Autodesk Inventor part; units mm, degrees
ref_plane "YZ Plane" through (0, 0, 0) normal (1, 0, 0) x (0, 1, 0)
ref_plane "XZ Plane" through (0, 0, 0) normal (0, 1, 0) x (-1, 0, 0)
ref_plane "XY Plane" through (0, 0, 0) normal (0, 0, 1) x (1, 0, 0)
sketch "Sketch1" plane through (0, 0, 0) normal (0, 0, 1) x (1, 0, 0)
  line L0 (3.6, -16) -> (3.6, 16)
  line L1 (-3.6, 16) -> (-3.6, -16)
  arc A0 (3.6, 16) -> (-3.6, 16) centre (0, 16) ccw
  circle A1 centre (0, 8) radius 2.4
  circle A2 centre (0, 8) radius 3.2
  circle A3 centre (0, 0) radius 3.2
  circle A4 centre (0, 0) radius 2.4
  line L2 (0, 0) -> (0, 8) construction
  line L3 (-2.8, 5.7373) -> (-2.8, 2.2627)
  line L4 (2.8, 5.7373) -> (2.8, 2.2627)
  arc A5 (-2.8, 5.7373) -> (2.8, 5.7373) centre (0, 8) ccw
  arc A6 (2.8, 2.2627) -> (-2.8, 2.2627) centre (0, 0) ccw
  arc A7 (-3.6, -16) -> (3.6, -16) centre (0, -16) ccw
  circle A8 centre (0, -8) radius 3.2
  circle A9 centre (0, -8) radius 2.4
  line L5 (0, 0) -> (0, -8) construction
  line L6 (-2.8, -2.2627) -> (-2.8, -5.7373)
  line L7 (2.8, -2.2627) -> (2.8, -5.7373)
  arc A10 (-2.8, -2.2627) -> (2.8, -2.2627) centre (0, 0) ccw
  arc A11 (2.8, -5.7373) -> (-2.8, -5.7373) centre (0, -8) ccw
  circle A12 centre (0, 16) radius 3.2
  circle A13 centre (0, 16) radius 2.4
  circle A14 centre (0, -16) radius 3.2
  circle A15 centre (0, -16) radius 2.4
  line L8 (0, 16) -> (0, 8) construction
  line L9 (0, -8) -> (0, -16) construction
  line L10 (2.8, 13.7373) -> (2.8, 10.2627)
  line L11 (-2.8, 13.7373) -> (-2.8, 10.2627)
  arc A16 (-2.8, 13.7373) -> (2.8, 13.7373) centre (0, 16) ccw
  arc A17 (2.8, 10.2627) -> (-2.8, 10.2627) centre (0, 8) ccw
  arc A18 (-2.8, -10.2627) -> (2.8, -10.2627) centre (0, -8) ccw
  arc A19 (2.8, -13.7373) -> (-2.8, -13.7373) centre (0, -16) ccw
  line L12 (2.8, -13.7373) -> (2.8, -10.2627)
  line L13 (-2.8, -10.2627) -> (-2.8, -13.7373)
  dimension "d8" = 4.8
  dimension "d9" = 6.4
  dimension "d32" = 7.2
  dimension "d34" = 8
  dimension "d36" = 0.8
extrude "Extrusion1" add sketch "Sketch1" along normal mid plane 8 contours A7 L1 A0 L0 | A2 | A3 | A5 L4 A6 L3 | A8 | A10 L7 A11 L6 | A12 | A14 | L10 A17 L11 A16 | A18 L12 A19 L13
sketch "Sketch6" plane through (0, 0, 4) normal (0, 0, 1) x (1, 0, 0)
  circle A0 centre (0, 0) radius 2.4
  circle A1 centre (0, 8) radius 2.4
  circle A2 centre (0, 0) radius 3.2
  circle A3 centre (0, 8) radius 3.2
  arc A4 (2.8, 2.2627) -> (-2.8, 2.2627) centre (0, 0) ccw
  line L0 (-2.8, 5.7373) -> (-2.8, 2.2627)
  arc A5 (-2.8, 5.7373) -> (2.8, 5.7373) centre (0, 8) ccw
  line L1 (2.8, 5.7373) -> (2.8, 2.2627)
  line L2 (-2.8, -2.2627) -> (-2.8, -5.7373)
  arc A6 (-2.8, -2.2627) -> (2.8, -2.2627) centre (0, 0) ccw
  arc A7 (2.8, -5.7373) -> (-2.8, -5.7373) centre (0, -8) ccw
  line L3 (2.8, -2.2627) -> (2.8, -5.7373)
  circle A8 centre (0, -8) radius 3.2
  circle A9 centre (0, -8) radius 2.4
  circle A10 centre (0, -16) radius 2.4
  circle A11 centre (0, 16) radius 2.4
  line L4 (2.8, -13.7373) -> (2.8, -10.2627)
  arc A12 (2.8, -13.7373) -> (-2.8, -13.7373) centre (0, -16) ccw
  arc A13 (-2.8, -10.2627) -> (2.8, -10.2627) centre (0, -8) ccw
  line L5 (-2.8, -10.2627) -> (-2.8, -13.7373)
  circle A14 centre (0, -16) radius 3.2
  circle A15 centre (0, 16) radius 3.2
  line L6 (2.8, 13.7373) -> (2.8, 10.2627)
  arc A16 (-2.8, 13.7373) -> (2.8, 13.7373) centre (0, 16) ccw
  arc A17 (2.8, 10.2627) -> (-2.8, 10.2627) centre (0, 8) ccw
  line L7 (-2.8, 13.7373) -> (-2.8, 10.2627)
extrude "Extrusion7" cut sketch "Sketch6" against normal blind 0.8 contours A2 | A3 | A8 | A14 | A15
extrude "Extrusion8" cut sketch "Sketch6" against normal blind 3.1 contours A4 L0 A5 L1 | A6 L3 A7 L2 | A12 L5 A13 L4 | L6 A17 L7 A16
mirror "Mirror1" about plane through (0, 0, 0) normal (0, 0, 1) of "Extrusion7", "Extrusion8"
fillet "Fillet1" radius 0.4 32 edges at (-2.8, 2.2627, 2.45) (-2.8, 5.7373, 2.45) (2.8, 2.2627, 2.45) (2.8, 5.7373, 2.45) (2.8, 5.7373, -2.45) (2.8, 2.2627, -2.45) (-2.8, 2.2627, -2.45) (-2.8, 5.7373, -2.45) (-2.8, -2.2627, 2.45) (-2.8, -5.7373, 2.45) (2.8, -5.7373, 2.45) (2.8, -2.2627, 2.45) (2.8, -2.2627, -2.45) (2.8, -5.7373, -2.45) (-2.8, -5.7373, -2.45) (-2.8, -2.2627, -2.45) (-2.8, -13.7373, 2.45) (-2.8, -13.7373, -2.45) (-2.8, -10.2627, 2.45) (-2.8, -10.2627, -2.45) (2.8, -13.7373, 2.45) (2.8, -10.2627, 2.45) (2.8, -13.7373, -2.45) (2.8, -10.2627, -2.45) (-2.8, 10.2627, 2.45) (-2.8, 13.7373, 2.45) (-2.8, 10.2627, -2.45) (-2.8, 13.7373, -2.45) (2.8, 10.2627, 2.45) (2.8, 13.7373, 2.45) (2.8, 10.2627, -2.45) (2.8, 13.7373, -2.45)
fillet "Fillet1" radius 0.1 8 edges at (0, -19.6, 4) (-3.6, 0, 4) (0, 19.6, 4) (3.6, 0, 4) (0, 19.6, -4) (-3.6, 0, -4) (0, -19.6, -4) (3.6, 0, -4)
equation "\"lf\" = 0.1"
equation "\"tf\" = 0.4"
properties part number "32316-DkBluishGray" material "ABS Plastic"
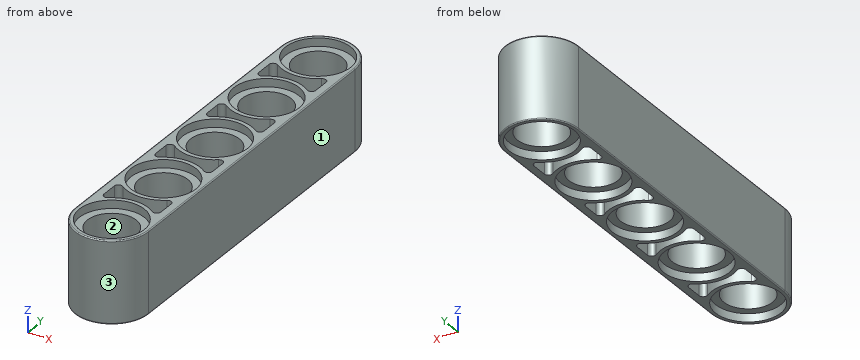
The model under review builds one solid part; all positions refer to its coordinate system, in mm. Face numbers are marked on the shaded views. Round coordinates to 2 decimals unless told otherwise and drop trailing zeros. Order: outer loops, then holes, each group sorted by start corner. A loop starts at its lowest first (then second) coordinate and runs counter-clockwise, first axis right, second up.
Item 1: For pin 1 (0.7 mm diameter, centred on x = 0.5, y = 12, fed in from +Z); pin 2 (3 mm diameter, centred on x = -1, y = -7, fed in from +Z); pin 3 (3 mm diameter, centred on x = -1, y = -7, fed in from -Z), all flat-tipped, find the tip position at first contact; note any pin that passes through.
Working result:
pin 1: stops at z = 0.9
pin 2: stops at z = 3.2
pin 3: stops at z = -3.2
Item 2: Add section D-D, the plane y = -9.5. State the section outline as (x, z) points.
Working result:
outline: (-3.6, -3.9) arc R0.1 ccw to (-3.5, -4) - (-2.83, -4) - (-2.83, -3.2) - (-1.87, -3.2) - (-1.87, 3.2) - (-2.83, 3.2) - (-2.83, 4) - (-3.5, 4) arc R0.1 ccw to (-3.6, 3.9) - close; (1.87, -3.2) - (2.83, -3.2) - (2.83, -4) - (3.5, -4) arc R0.1 ccw to (3.6, -3.9) - (3.6, 3.9) arc R0.1 ccw to (3.5, 4) - (2.83, 4) - (2.83, 3.2) - (1.87, 3.2) - close
Item 3: Add section A-A, the plane y = 0. State the section outline as (x, z) points.
Working result:
outline: (-3.6, -3.9) arc R0.1 ccw to (-3.5, -4) - (-3.2, -4) - (-3.2, -3.2) - (-2.4, -3.2) - (-2.4, 3.2) - (-3.2, 3.2) - (-3.2, 4) - (-3.5, 4) arc R0.1 ccw to (-3.6, 3.9) - close; (2.4, -3.2) - (3.2, -3.2) - (3.2, -4) - (3.5, -4) arc R0.1 ccw to (3.6, -3.9) - (3.6, 3.9) arc R0.1 ccw to (3.5, 4) - (3.2, 4) - (3.2, 3.2) - (2.4, 3.2) - close
Item 4: To check wall thickness, follow probe 1 along Y at (x, z) = (-0.75, 0.25); probe 2 along Z at (x, y) = (1.5, -2.5); probe 3 along Y at (x, z) = (1, 0.25). State the ranges of each line that lie inside material, in increasing order.
Working result:
probe 1: y = -19.52 to -18.28, -13.72 to -10.28, -5.72 to -2.28, 2.28 to 5.72, 10.28 to 13.72, 18.28 to 19.52
probe 2: z = -3.2 to 3.2
probe 3: y = -19.46 to -18.18, -13.82 to -10.18, -5.82 to -2.18, 2.18 to 5.82, 10.18 to 13.82, 18.18 to 19.46
Item 5: Add section C-C, the plane x = 0. Count the separate pieces of the cut face and the enclosed holes in it, and give its area (4 significant figures).
Working result:
separate pieces: 6
enclosed holes: 0
area: 88.95 mm2
Item 6: Draft analysis for pull direction Y (two halves, no side actions). For the marked faces 1, 2 and 3, state which applies: released by +Y, released by -Y, zero draft, split by the parting line, or undercut.
Working result:
face 1: zero draft
face 2: undercut
face 3: released by -Y
Item 7: Add section B-B, the plane z = 0.5. State the section outline as (x, y) points.
Working result:
outline: (-3.6, -16) arc R3.6 ccw to (3.6, -16) - (3.6, 16) arc R3.6 ccw to (-3.6, 16) - close; hole circle Ø4.8 at (0, -16); hole circle Ø4.8 at (0, -8); hole circle Ø4.8 at (0, 0); hole circle Ø4.8 at (0, 8); hole circle Ø4.8 at (0, 16)
